Geometry check sheet. Reference: the model listing, model coordinates, mm. A direction names the side the tool comes from. Coordinates: 2 decimals unless noted, no trailing zeros. Write each loop counter-clockwise with the first axis right and the second up, starting at its lowest first coordinate (ties: lowest second). Pieces come first, ordered by that corner, then holes. Notation, with made-up numbers: (27, -23) -> (33, -23) arc R16 cw to (33, -6) -> close; hole circle Ø6 at (49.5, 30.25). An arc over 180 degrees is marked (long way). Use a Markdown table: item, result.
```python
from build123d import *

# Parameters (mm, degrees)
CROQUIS1_W              = 8
CROQUIS1_H              = 25.6
CROQUIS1_R              = 1.5
SALIENTE_EXTRUIR1_DEPTH = 6
REDONDEO1_R             = 4
CROQUIS2_R              = 3
CORTAR_EXTRUIR1_DEPTH   = 2
CROQUIS3_R              = 2.8
CORTAR_EXTRUIR2_DEPTH   = 8


with BuildPart() as part:
    # Croquis1 → Saliente-Extruir1 (new body)
    with BuildSketch(Plane.XY):
        with Locations((-128.440920984, 53.999185999)):
            Rectangle(CROQUIS1_W, CROQUIS1_H)
        with Locations((-128.440920984, 61.799185999)):
            Circle(CROQUIS1_R, mode=Mode.SUBTRACT)
        with Locations((-128.440920984, 46.199185999)):
            Circle(CROQUIS1_R, mode=Mode.SUBTRACT)
    extrude(amount=SALIENTE_EXTRUIR1_DEPTH)

    # Redondeo1
    # the kernel refuses this fillet: 4 mm, written as the material it takes off along each edge
    with BuildSketch(Plane(origin=(-142.440920984, 66.799185999, 6), x_dir=(0, 0, -1), z_dir=(1, 0, 0)), Plane(origin=(-114.440920984, 41.199185999, 6), x_dir=(0, 0, -1), z_dir=(-1, 0, 0))) as redondeo1_piece_1:
        with BuildLine():
            CenterArc((REDONDEO1_R, -REDONDEO1_R), REDONDEO1_R, 90, 90)
            Line((0, -REDONDEO1_R), (0, 0))
            Line((0, 0), (REDONDEO1_R, 0))
        make_face()
    extrude(amount=28, mode=Mode.SUBTRACT)

    # Croquis2 → Cortar-Extruir1 (cut)
    with BuildSketch(Plane.XY.offset(6)):
        with Locations((-128.440920984, 46.199185999)):
            Circle(CROQUIS2_R)
        with Locations((-128.440920984, 61.799185999)):
            Circle(CROQUIS2_R)
    extrude(amount=-CORTAR_EXTRUIR1_DEPTH, mode=Mode.SUBTRACT)

    # Croquis3 → Cortar-Extruir2 (cut)
    with BuildSketch(Plane(origin=(-124.440920984, 0, 0), x_dir=(0, 0, -1), z_dir=(1, 0, 0))):
        with Locations((0, 53.999185999)):
            Circle(CROQUIS3_R)
    extrude(amount=-CORTAR_EXTRUIR2_DEPTH, mode=Mode.SUBTRACT)


solid = part.part
```
Item 1: Section check A-A on z = 2.5. Record the boundary of the cut face in (x, y), then the cut area to 3 significant figures.
Answer block:
| item | result |
|---|---|
| outline | (-132.44, 41.23) -> (-124.44, 41.23) -> (-124.44, 52.74) -> (-132.44, 52.74) -> close; (-132.44, 55.26) -> (-124.44, 55.26) -> (-124.44, 66.77) -> (-132.44, 66.77) -> close; hole circle Ø3 at (-128.44, 46.2); hole circle Ø3 at (-128.44, 61.8) |
| area | 170 mm^2 |
Item 2: Depth check by flat-ended pin: P1, Ø1.8, axis at x = -129.5, y = 61, coming from the +Z side; P2, Ø2, axis at x = -126.5, z = 4.5, coming from the -Y side. Enter the tip coordinate at first touch or a pass-through.
Answer block:
| item | result |
|---|---|
| P1 | stops at z = 4 |
| P2 | stops at y = 41.49 |
Item 3: Section check C-C on x = -126.5. Record the boundary of the cut face in (y, z).
Answer block:
| item | result |
|---|---|
| outline | (41.2, 0) -> (51.2, 0) arc R2.8 cw to (56.8, 0) -> (66.8, 0) -> (66.8, 2) arc R4 ccw to (64.09, 5.79) -> (64.09, 4) -> (59.51, 4) -> (59.51, 6) -> (48.49, 6) -> (48.49, 4) -> (43.91, 4) -> (43.91, 5.79) arc R4 ccw to (41.2, 2) -> close |
Item 4: Mould release check, pull along X, two halves, no side actions. Record for faces 3 (the cylindrical face through (-128.831, 49.174, 5.014)), 4 (the cylindrical face through (-128.4, 54.1, 2.8)), 5 (the flat face through (-124.441, 54, 3)), 6 (the flat face through (-132.441, 54, 3)): +X half, -X half, draft (parallel to the pull), parting line (faces both ways), or undercut.
Answer block:
| item | result |
|---|---|
| face 3 | undercut |
| face 4 | draft |
| face 5 | +X half |
| face 6 | -X half |
Item 5: Section check D-D on z = 3.75. Record the boundary of the cut face in (x, y).
Answer block:
| item | result |
|---|---|
| outline | (-132.44, 41.6) -> (-124.44, 41.6) -> (-124.44, 66.4) -> (-132.44, 66.4) -> close; hole circle Ø3 at (-128.44, 46.2); hole circle Ø3 at (-128.44, 61.8) |
Item 6: Section check B-B on x = -129.5. Record the boundary of the cut face in (y, z).
Answer block:
| item | result |
|---|---|
| outline | (41.2, 0) -> (45.14, 0) -> (45.14, 4) -> (43.39, 4) -> (43.39, 5.57) arc R4 ccw to (41.2, 2) -> close; (47.26, 0) -> (51.2, 0) arc R2.8 cw to (56.8, 0) -> (60.74, 0) -> (60.74, 4) -> (58.99, 4) -> (58.99, 6) -> (49.01, 6) -> (49.01, 4) -> (47.26, 4) -> close; (62.86, 0) -> (66.8, 0) -> (66.8, 2) arc R4 ccw to (64.61, 5.57) -> (64.61, 4) -> (62.86, 4) -> close |
Item 7: Thickness scan on L1, parallel to Y at x = -129.25, z = 3; L2, parallel to Y at x = -128, z = 1.25; L3, parallel to Y at x = -129.75, z = 2. Record the ranges inside material, lowest first. Write a range as [from, to].
Answer block:
| item | result |
|---|---|
| L1 | y = [41.33, 44.94], [47.46, 60.54], [63.06, 66.67] |
| L2 | y = [41.2, 44.77], [47.63, 51.49], [56.5, 60.37], [63.23, 66.8] |
| L3 | y = [41.2, 45.47], [46.93, 52.04], [55.96, 61.07], [62.53, 66.8] |
Item 8: Tool access check on faces 1 (the cylindrical face through (-129.09, 58.87, 5.01)), 2 (the flat face through (-130.3, 46.3, 0)). Record the directions out of +Z, -Z, +X, -X, +Y, -Y that give a thin tool (end or side, any length) a straight path to the whole face; none if there is none.
Answer block:
| item | result |
|---|---|
| face 1 | +Z |
| face 2 | -Z, +X, -X, +Y, -Y |
